Here's the drawing with two shaded views (mm, measured from the low corner). I have some questions. A direction names the side the tool comes from. Coordinates: 2 decimals unless noted, no trailing zeros. Loops run counter-clockwise (first coordinate to the right, second up) from the corner with the lowest first, then second, coordinate; pieces in that order, holes last. Notation, with made-up numbers: M 80,32.5 L 122,32.5 A21 cw 122,54.5 Z; hole C 53,6 d10. An arc over 180 degrees is marked long. Return JSON: item names as keys, results as strings. Group by question number.
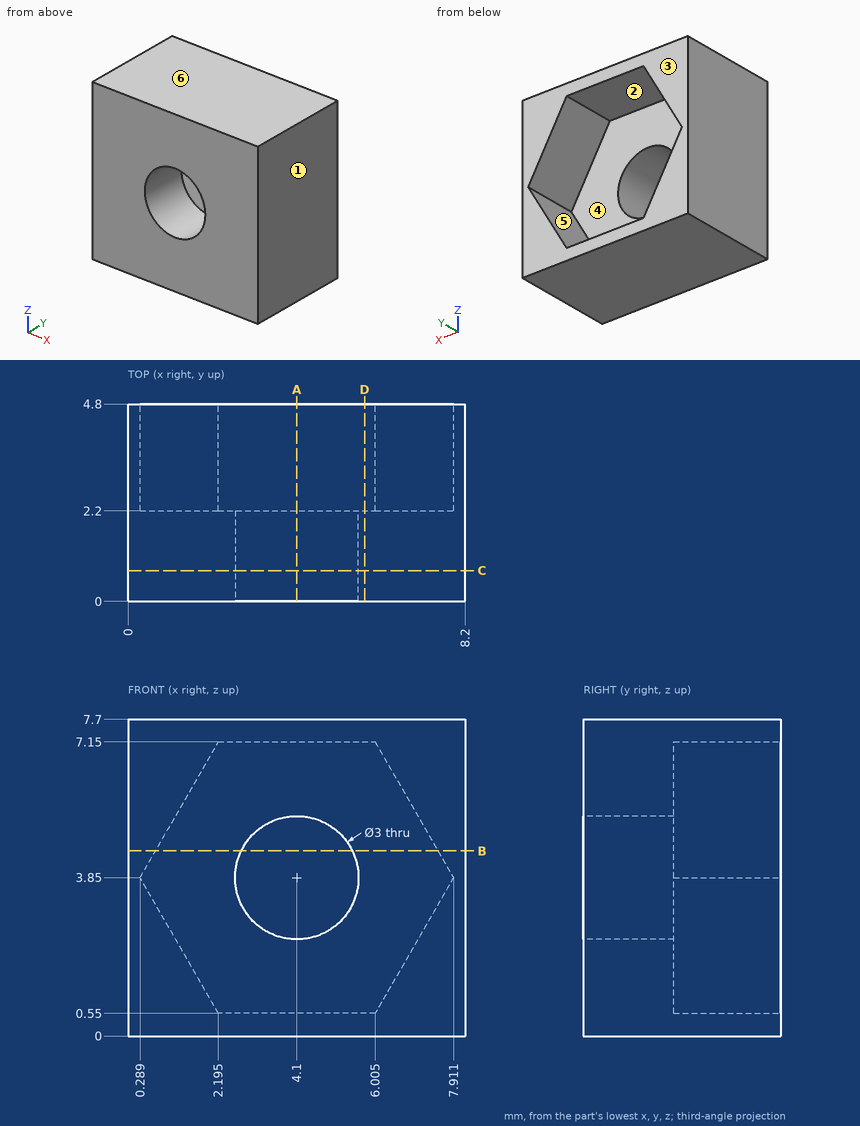
(1) If I drill on L1, parallel to Z at x = 4.1, y = 1.45; L2, parallel to X at y = 1.75, z = 3.85; L3, parallel to Y at x = 2.25, z = 2.75, over which ranges is the centre line in solid material (lowest first)? Write a range as [from, to].
(2) For the marked faces 1 and 2, which set-ups out of +Z, -Z, +X, -X, +Y, -Y let a thin tool reach every point of the face, with its end or its side?
(3) Will these pins go through, and if not, where does the flat tip stop? P1, Ø3.5, axis at x = 4.5, z = 2.5, coming from the +Y side; P2, Ø1, axis at x = 5, z = 2, coming from the -Y side.
(4) Imagine slicing it at D-D, the plane x = 5.75. Write out the boundary of the cut face in (y, z).
(5) We'd pull the mould along Z, two halves only. Please class the marked faces 3, 4, 5 and 6: +Z half, -Z half, draft (parallel to the pull), parting line (faces both ways), or undercut.
(6) Imagine slicing it at B-B, the plane z = 4.5. Write out the boundary of the cut face in (x, y) (1 decimal).
(7) Imagine slicing it at C-C, the plane y = 0.75. Write out the boundary of the cut face in (x, z).
(8) Imagine slicing it at A-A, the plane x = 4.1. Write out the boundary of the cut face in (y, z).
Checks:
{
 "1": {"L1": "[0, 2.35], [5.35, 7.7]", "L2": "[0, 2.6], [5.6, 8.2]", "L3": "[0, 2.2]"},
 "2": {"face 1": "+Z, -Z, +X, +Y, -Y", "face 2": "+Y"},
 "3": {"P1": "y = 2.2", "P2": "y = 0"},
 "4": {"outline": "M 0,0 L 4.8,0 L 4.8,0.55 L 2.2,0.55 L 2.2,7.15 L 4.8,7.15 L 4.8,7.7 L 0,7.7 Z"},
 "5": {"face 3": "draft", "face 4": "undercut", "face 5": "undercut", "face 6": "+Z half"},
 "6": {"outline": "M 0,0 L 2.7,0 L 2.7,2.2 L 0.7,2.2 L 0.7,4.8 L 0,4.8 Z; M 5.5,0 L 8.2,0 L 8.2,4.8 L 7.5,4.8 L 7.5,2.2 L 5.5,2.2 Z"},
 "7": {"outline": "M 0,0 L 8.2,0 L 8.2,7.7 L 0,7.7 Z; hole C 4.1,3.85 d3"},
 "8": {"outline": "M 0,0 L 4.8,0 L 4.8,0.55 L 2.2,0.55 L 2.2,2.35 L 0,2.35 Z; M 0,5.35 L 2.2,5.35 L 2.2,7.15 L 4.8,7.15 L 4.8,7.7 L 0,7.7 Z"}
}
